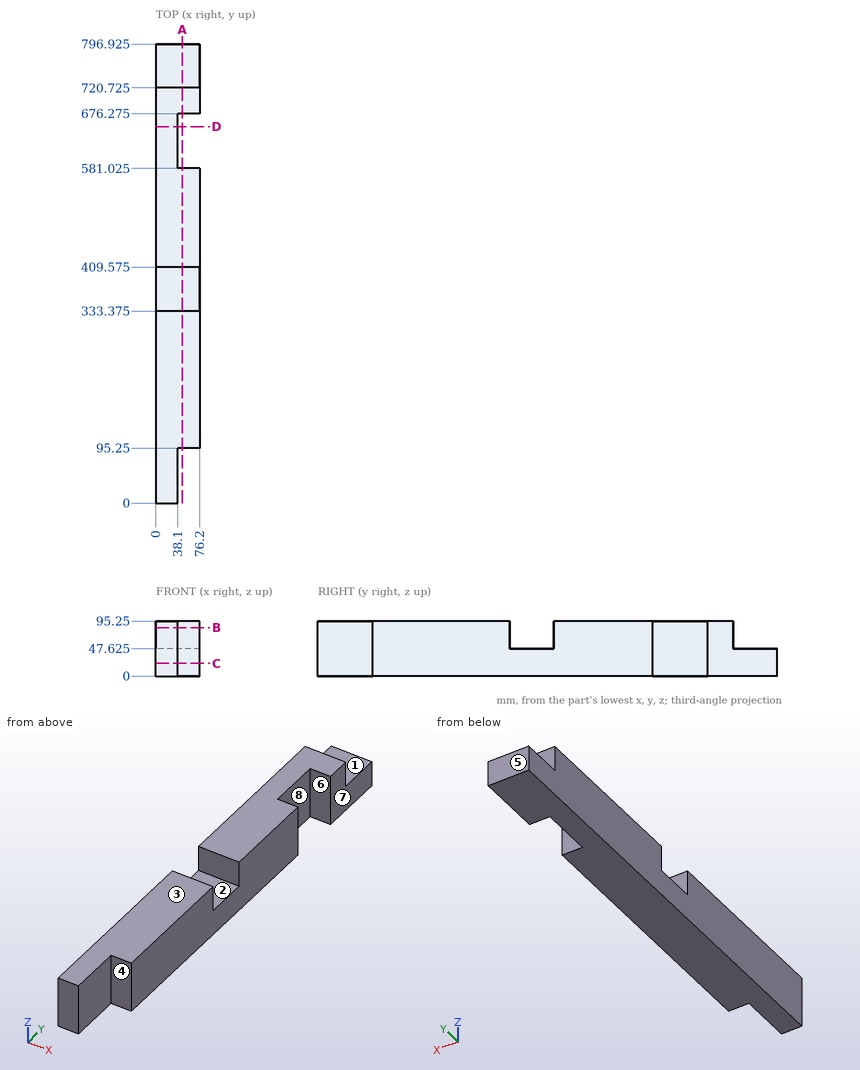
Verification items for this drawing (mm, ordinates from the low corner). A direction names the side the tool comes from. Round coordinates to 2 decimals unless told otherwise and drop trailing zeros. Loops run counter-clockwise (first coordinate to the right, second up) from the corner with the lowest first, then second, coordinate; pieces in that order, holes last. Notation, with made-up numbers: M -27,67 L -22,67 A13 ccw -22,72 Z; hole C 15.25,-19 d7. An arc over 180 degrees is marked long. Answer as a JSON object with one key per item and string values.
1. Mould release check, pull along Y, two halves, no side actions. Record for the marked faces 5, 6, 7 and 8: pulls with the +Y half, pulls with the -Y half, needs draft (parallel to the pull), parting line crosses it, or undercut.
Reply:
{"face 5": "pulls with the +Y half", "face 6": "undercut", "face 7": "needs draft", "face 8": "undercut"}
2. Section check A-A (x = 46). Record the boundary of the cut face in (y, z) (3 decimals), plus the area to 3 significant figures.
Reply:
{"outline": "M 95.25,0 L 581.025,0 L 581.025,95.25 L 409.575,95.25 L 409.575,47.625 L 333.375,47.625 L 333.375,95.25 L 95.25,95.25 Z; M 676.275,0 L 796.925,0 L 796.925,47.625 L 720.725,47.625 L 720.725,95.25 L 676.275,95.25 Z", "area": "50,500 mm²"}
3. Gauge pin test, flat ends, axial feed: P1, Ø24, axis at x = 29.5, z = 64, coming from the +Y side (3 decimals); P2, Ø2, axis at x = 47.5, z = 67, coming from the -Y side. Record the tip position at first contact, or that the pin passes through.
Reply:
{"P1": "stops at y = 720.725", "P2": "stops at y = 95.25"}
4. Section check D-D (y = 653.5). Record the boundary of the cut face in (x, z), plus the area to 3 significant figures.
Reply:
{"outline": "M 0,0 L 38.1,0 L 38.1,95.25 L 0,95.25 Z", "area": "3,630 mm²"}
5. Section check C-C (z = 22). Record the boundary of the cut face in (x, y) (3 decimals), plus the area to 3 significant figures.
Reply:
{"outline": "M 0,0 L 38.1,0 L 38.1,95.25 L 76.2,95.25 L 76.2,581.025 L 38.1,581.025 L 38.1,676.275 L 76.2,676.275 L 76.2,796.925 L 0,796.925 Z", "area": "53,500 mm²"}
6. Access from +Z, -Z, +X, -X, +Y, -Y to the whole of each face (thin tool, end or side, straight path). Record for the marked faces 1, 2, 3 and 4.
Reply:
{"face 1": "+Z, +X, -X, +Y", "face 2": "+Z, +X, -X", "face 3": "+Z, +X, -X, +Y, -Y", "face 4": "+Z, -Z, +X, -Y"}
7. Scan lines: line 1 (Y direction, x = 9.5, z = 83) (3 decimals); line 2 (Y direction, x = 60.5, z = 18.5) (3 decimals); line 3 (X direction, y = 583.5, z = 81.5). Record each from-to range of solid material in increasing order.
Reply:
{"line 1": "y = 0 to 333.375, 409.575 to 720.725", "line 2": "y = 95.25 to 581.025, 676.275 to 796.925", "line 3": "x = 0 to 38.1"}
8. Section check B-B (z = 84). Record the boundary of the cut face in (x, y) (3 decimals).
Reply:
{"outline": "M 0,0 L 38.1,0 L 38.1,95.25 L 76.2,95.25 L 76.2,333.375 L 0,333.375 Z; M 0,409.575 L 76.2,409.575 L 76.2,581.025 L 38.1,581.025 L 38.1,676.275 L 76.2,676.275 L 76.2,720.725 L 0,720.725 Z"}
